Study the drawing (mm; zero at the part's minimum x, y, z) and answer. Round coordinates to 2 decimals unless told otherwise and drop trailing zeros. Loops run counter-clockwise (first coordinate to the right, second up) from the corner with the lowest first, then second, coordinate; pieces in that order, holes last. Notation, with made-up numbers: (12, 16) -> (67, 16) arc R21 cw to (67, 46) -> close; hole circle Ø8 at (71, 39.25). An arc over 180 degrees is marked (long way). Write each question's results on one line, items separated by ' | '. Start each with the question number.
(1) The part is cut by section A-A (z = 6). Determine the outline of the cut face in (x, y).
(2) Straight lines are drawn through the part: probe 1 along X at (y, z) = (2.9, 7.5); probe 2 along Z at (x, y) = (129.6, 1.45); probe 3 along X at (y, z) = (1.85, 5.5). For each, find the intervals that lie inside material, in ascending order.
(3) A flat-ended cylindrical pin translates along its axis: pin 1 (1.5 mm diameter, centred on y = 3, z = 3.5, fed in from -X). Find the tip coordinate at first contact, or state that the pin passes through.
(4) The part is cut by section B-B (x = 30). Determine the outline of the cut face in (y, z).
(5) The part is cut by section C-C (y = 2.15). Determine the outline of the cut face in (x, z), plus the area to 3 significant figures.
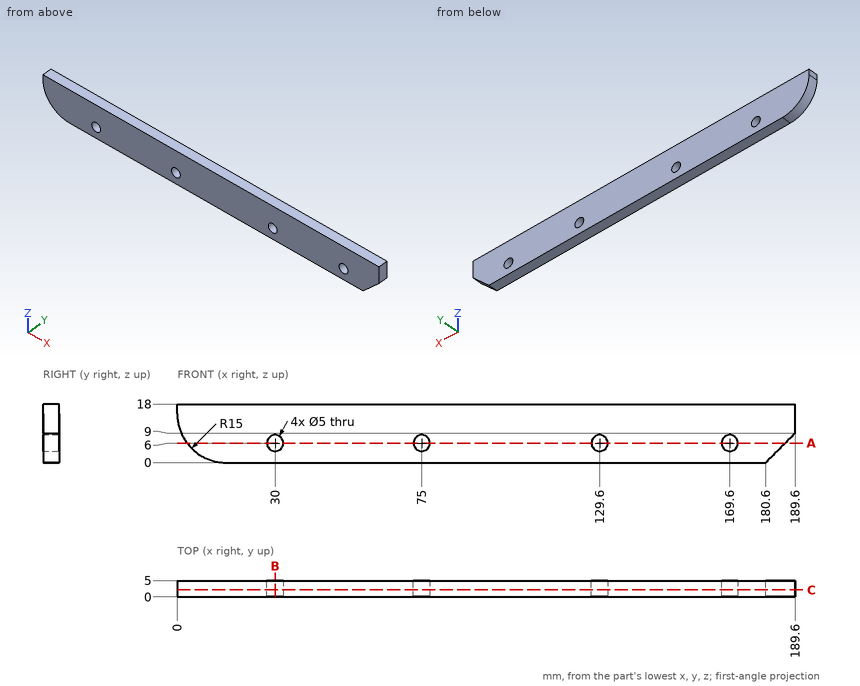
Checked values:
1) outline: (3, 0) -> (27.5, 0) -> (27.5, 5) -> (3, 5) -> close; (32.5, 0) -> (72.5, 0) -> (72.5, 5) -> (32.5, 5) -> close; (77.5, 0) -> (127.1, 0) -> (127.1, 5) -> (77.5, 5) -> close; (132.1, 0) -> (167.1, 0) -> (167.1, 5) -> (132.1, 5) -> close; (172.1, 0) -> (186.6, 0) -> (186.6, 5) -> (172.1, 5) -> close
2) probe 1: x = 2.01 to 28, 32 to 73, 77 to 127.6, 131.6 to 167.6, 171.6 to 188.1 | probe 2: z = 0 to 3.5, 8.5 to 18 | probe 3: x = 3.39 to 27.55, 32.45 to 72.55, 77.45 to 127.15, 132.05 to 167.15, 172.05 to 186.1
3) pin 1: stops at x = 4.54
4) outline: (0, 0) -> (5, 0) -> (5, 3.5) -> (0, 3.5) -> close; (0, 8.5) -> (5, 8.5) -> (5, 18) -> (0, 18) -> close
5) outline: (0, 15) arc R15 ccw to (15, 0) -> (180.6, 0) -> (189.6, 9) -> (189.6, 18) -> (0, 18) -> close; hole circle Ø5 at (30, 6); hole circle Ø5 at (75, 6); hole circle Ø5 at (129.6, 6); hole circle Ø5 at (169.6, 6) | area: 3,250 mm2
